from build123d import *

# Parameters (mm, degrees)
SKETCH_1_W           = 7.62
SKETCH_1_H           = 2.54
EXTRUDE_1_DEPTH      = 2.54
EXTRUDE_2_DEPTH      = 6
EXTRUDE_2_DEPTH_BACK = 5
SKETCH_2_R           = 0.4


with BuildPart() as part:
    # Sketch 1 → Extrude 1 (new body)
    with BuildSketch(Plane.XY):
        with Locations((3.81, 1.27)):
            Rectangle(SKETCH_1_W, SKETCH_1_H)
    extrude(amount=EXTRUDE_1_DEPTH)

    # Sketch 2 → Extrude 2 (add, two sides: drawn at the far end of the back side and taken through both)
    with BuildSketch(Plane.XY.offset(2.54).offset(-EXTRUDE_2_DEPTH_BACK)):
        with Locations(Location((1.174408602, 1.27, 0), (0, 0, 180))):
            Circle(SKETCH_2_R)
        with Locations(Location((3.714408602, 1.27, 0), (0, 0, 180))):
            Circle(SKETCH_2_R)
        with Locations(Location((6.254408602, 1.27, 0), (0, 0, 180))):
            Circle(SKETCH_2_R)
    extrude(amount=EXTRUDE_2_DEPTH + EXTRUDE_2_DEPTH_BACK)


solid = part.part
Design review of the part built by this model. Coordinates are the model's own, in mm. A direction names the side the tool comes from. Give positions to 0.01 mm unless a question says otherwise; leave off trailing zeros. Write each loop counter-clockwise with the first axis right and the second up, starting at its lowest first coordinate (ties: lowest second). Pieces come first, ordered by that corner, then holes. Notation, with made-up numbers: M 17,22 L 22,22 A36 ccw 22,56 Z; hole C 86,31 d11. An arc over 180 degrees is marked long. Answer as a JSON object with one key per item and string values. Group by question number.
1) We need section C-C (x = 1). Give the boundary of the cut face in (y, z).
2) For line 1 along X through (y, z) = (1.4, 7.5); line 2 along Z through (x, y) = (7, 1.2); line 3 along X through (y, z) = (0.95, 7.5), list the stretches that pass through material, from the lowest coordinate up.
3) We need section B-B (y = 1.27). Give the boundary of the cut face in (x, z).
4) We need section A-A (z = 6.25). Give the boundary of the cut face in (x, y), and give its area (3 significant figures).
5) Mouldability with a two-part tool opening along X and no side actions: class faces 1 (the face through (0, 1, 1)), 2 (the face through (4, 0, 1)), 3 (the face through (3.345, 1.423, -1.247)) as released by +X, released by -X, zero draft, split by the parting line, or undercut.
6) We need section D-D (y = 0.6). Give the boundary of the cut face in (x, z).
7) Clearance check with flat-ended pins moving along their axes: pin 1 Ø1 at (y, z) = (0.5, 1) entering from -X; pin 2 Ø1.3 at (x, y) = (5, 1.5) entering from -Z; pin 3 Ø1 at (y, z) = (0.5, 5.5) entering from +X; pin 4 Ø3 at (x, z) = (4, 6.5) entering from +Y. State where each tip first meets the part, or that it passes through.
8) Tool access review of faces 4 (the face through (7.62, 1, 1)), 5 (the face through (6.572, 1.513, -1.247)), 6 (the face through (3.345, 1.423, 5.498)): name each direction out of +Z, -Z, +X, -X, +Y, -Y from which nothing blocks a thin tool from reaching the whole face with its end or side.
Answer key:
{
 "1": {"outline": "M 0,0 L 0.91,0 L 0.91,-2.46 L 1.63,-2.46 L 1.63,0 L 2.54,0 L 2.54,2.54 L 1.63,2.54 L 1.63,8.54 L 0.91,8.54 L 0.91,2.54 L 0,2.54 Z"},
 "2": {"line 1": "x = 0.8 to 1.55, 3.34 to 4.09, 5.88 to 6.63", "line 2": "z = 0 to 2.54", "line 3": "x = 0.93 to 1.41, 3.47 to 3.95, 6.01 to 6.49"},
 "3": {"outline": "M 0,0 L 0.77,0 L 0.77,-2.46 L 1.57,-2.46 L 1.57,0 L 3.31,0 L 3.31,-2.46 L 4.11,-2.46 L 4.11,0 L 5.85,0 L 5.85,-2.46 L 6.65,-2.46 L 6.65,0 L 7.62,0 L 7.62,2.54 L 6.65,2.54 L 6.65,8.54 L 5.85,8.54 L 5.85,2.54 L 4.11,2.54 L 4.11,8.54 L 3.31,8.54 L 3.31,2.54 L 1.57,2.54 L 1.57,8.54 L 0.77,8.54 L 0.77,2.54 L 0,2.54 Z"},
 "4": {"outline": "C 1.17,1.27 d0.8; C 3.71,1.27 d0.8; C 6.25,1.27 d0.8", "area": "1.51 mm²"},
 "5": {"face 1": "released by -X", "face 2": "zero draft", "face 3": "undercut"},
 "6": {"outline": "M 0,0 L 7.62,0 L 7.62,2.54 L 0,2.54 Z"},
 "7": {"pin 1": "stops at x = 0", "pin 2": "stops at z = 0", "pin 3": "stops at x = 6.55", "pin 4": "stops at y = 1.67"},
 "8": {"face 4": "+Z, -Z, +X, +Y, -Y", "face 5": "-Z", "face 6": "+Z"}
}
